For this review, use the dimensioned drawing (mm, ordinates from the lowest corner) and the shaded views. A direction names the side the tool comes from. Give positions to 0.01 mm unless a question says otherwise; leave off trailing zeros. Write each loop counter-clockwise with the first axis right and the second up, starting at its lowest first coordinate (ties: lowest second). Pieces come first, ordered by that corner, then holes. Notation, with made-up numbers: (35, -36.5) -> (83, -36.5) arc R34 ccw to (83, -1.5) -> close; hole circle Ø3 at (-28.75, 9.25). An arc over 180 degrees is marked (long way). Answer as CSV lines item,"result".
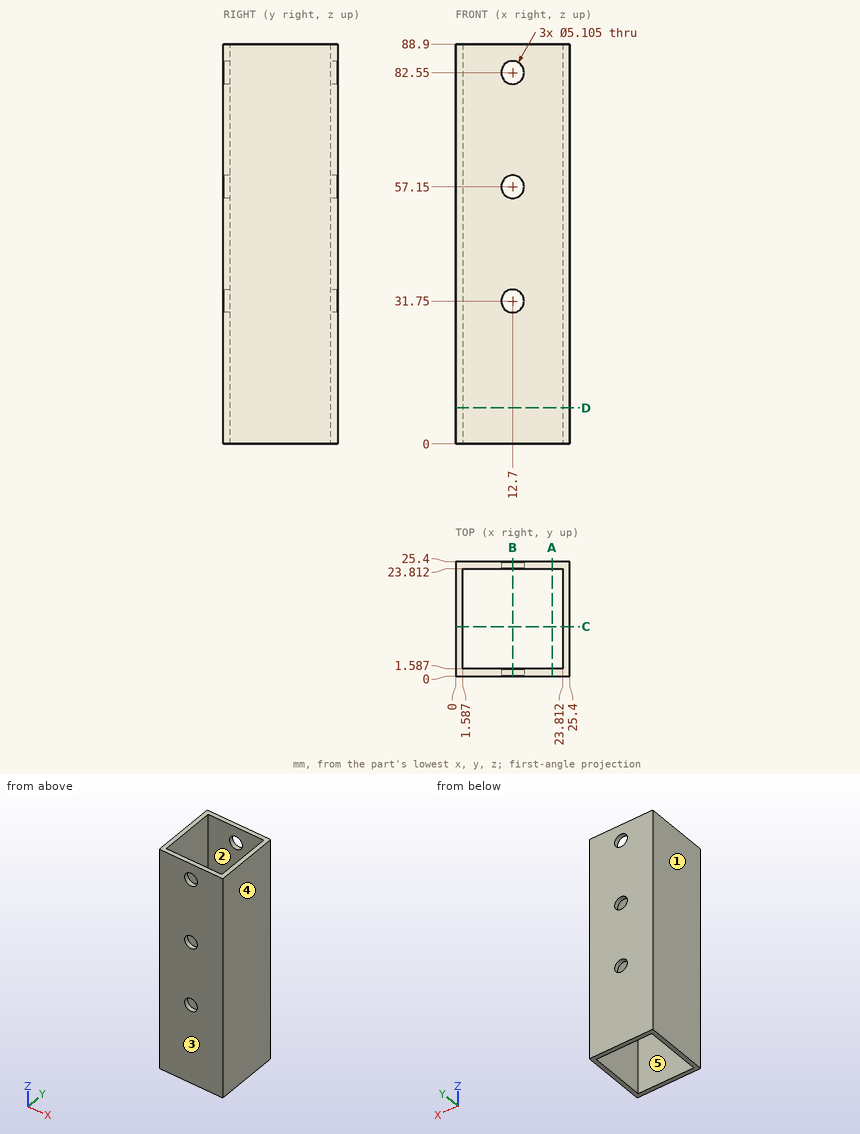
Q1. Add section A-A (x = 21.5). Write out the cut boundary in (y, z).
Answer block:
outline,"(0, 0) -> (1.59, 0) -> (1.59, 88.9) -> (0, 88.9) -> close; (23.81, 0) -> (25.4, 0) -> (25.4, 88.9) -> (23.81, 88.9) -> close"
Q2. For the marked faces 1 and 2, list the 3-axis set-ups (+Z, -Z, +X, -X, +Y, -Y) from which the entire face can be reached by the end or side of a thin tool; tool diameter is ignored.
Answer block:
face 1,"+Z, -Z, -X, +Y, -Y"
face 2,"+Z, -Z"
Q3. To check wall thickness, follow probe 1 along Z at (x, y) = (12.7, 0.95); probe 2 along X at (y, z) = (0.6, 82.55); probe 3 along Y at (x, z) = (4, 52). State the ranges of each line that lie inside material, in increasing order. Write a range as [from, to].
Answer block:
probe 1,"z = [0, 29.2], [34.3, 54.6], [59.7, 80], [85.1, 88.9]"
probe 2,"x = [0, 10.15], [15.25, 25.4]"
probe 3,"y = [0, 1.59], [23.81, 25.4]"
Q4. Draft analysis for pull direction X (two halves, no side actions). For the marked faces 3, 4 and 5, state which applies: released by +X, released by -X, zero draft, split by the parting line, or undercut.
Answer block:
face 3,"zero draft"
face 4,"released by +X"
face 5,"undercut"
Q5. Add section D-D (z = 8). Write out the cut boundary in (x, y).
Answer block:
outline,"(0, 0) -> (25.4, 0) -> (25.4, 25.4) -> (0, 25.4) -> close; hole (1.59, 1.59) -> (23.81, 1.59) -> (23.81, 23.81) -> (1.59, 23.81) -> close"
Q6. Add section B-B (x = 12.7). State how many separate pieces and enclosed holes the cut face has.
Answer block:
separate pieces,"8"
enclosed holes,"0"
